The listing builds one solid part. Answer for the finished solid, in the listing's coordinates (mm). A direction names the side the tool comes from. Round coordinates to 2 decimals unless told otherwise and drop trailing zeros. Loops run counter-clockwise (first coordinate to the right, second up) from the corner with the lowest first, then second, coordinate; pieces in that order, holes last. Notation, with made-up numbers: (67, 76) -> (99, 76) arc R12 cw to (99, 98) -> close; hole circle Ø5 at (81, -5). An arc over 180 degrees is marked (long way). Answer in a Markdown table with one row per item. Add a question column.
```python
from build123d import *

# Parameters (mm, degrees)
SKETCH2_R                     = 3.811725635
F_18_TEETH_KNURLS_DEPTH       = 5.9944
SKETCH3_W                     = 1
SKETCH3_H                     = 6.35
CUT_EXTRUDE2_DEPTH            = 5.9944
SKETCH4_W                     = 9.4996
SKETCH4_H                     = 11.303
BODY_DEPTH                    = 7.0612
SKETCH6_W                     = 0.2286
SKETCH6_H                     = 0.7874
PINS_PTD901_ONE_SECTION_DEPTH = 3.5


with BuildPart() as part:
    # Sketch1 → Shaft Base (revolve)
    with BuildSketch(Plane.XY):
        Polygon((0, 3.5), (4.52755, 3.5), (5.0038, 3.02375), (5.0038, 0), (0, 0), align=None)
    revolve(axis=Axis((-1.517556918, 0, 0), (1, 0, 0)))

    # Sketch8 → K Style Shaft (revolve)
    with BuildSketch(Plane.XY):
        Polygon((5.0038, 3.00589629), (5.0038, 0), (15, 0), (15, 2.01414629), (14.0348, 2.97934629), (9.0056, 2.97934629), (9.0056, 2.01414629), (6.5024, 2.01414629), (5.51065, 3.00589629), align=None)
    revolve(axis=Axis((-8.258778459, 0, 0), (1, 0, 0)))

    # Sketch2 → 18 Teeth Knurls (cut)
    with BuildSketch(Plane(origin=(15, 0, 0), x_dir=(0, 0, -1), z_dir=(1, 0, 0))):
        Circle(SKETCH2_R)
        Polygon((0, 2.97934629), (0.353893751, 2.007031199), (1.018996445, 2.799669723), (1.018996445, 1.764953616), (1.91508688, 2.282311669), (1.561193129, 1.309996578), (2.580189574, 1.489673145), (1.91508688, 0.69703462), (2.934083325, 0.517358054), (2.03799289, 0), (2.934083325, -0.517358054), (1.91508688, -0.69703462), (2.580189574, -1.489673145), (1.561193129, -1.309996578), (1.91508688, -2.282311669), (1.018996445, -1.764953616), (1.018996445, -2.799669723), (0.353893751, -2.007031199), (0, -2.97934629), (-0.353893751, -2.007031199), (-1.018996445, -2.799669723), (-1.018996445, -1.764953616), (-1.91508688, -2.282311669), (-1.561193129, -1.309996578), (-2.580189574, -1.489673145), (-1.91508688, -0.69703462), (-2.934083325, -0.517358054), (-2.03799289, 0), (-2.934083325, 0.517358054), (-1.91508688, 0.69703462), (-2.580189574, 1.489673145), (-1.561193129, 1.309996578), (-1.91508688, 2.282311669), (-1.018996445, 1.764953616), (-1.018996445, 2.799669723), (-0.353893751, 2.007031199), align=None, mode=Mode.SUBTRACT)
    extrude(amount=-F_18_TEETH_KNURLS_DEPTH, mode=Mode.SUBTRACT)

    # Sketch3 → Cut-Extrude2 (cut)
    with BuildSketch(Plane(origin=(15, 0, 0), x_dir=(0, 0, -1), z_dir=(1, 0, 0))):
        Rectangle(SKETCH3_W, SKETCH3_H)
    extrude(amount=-CUT_EXTRUDE2_DEPTH, mode=Mode.SUBTRACT)

    # Sketch4 → Body (add)
    with BuildSketch(Plane.ZY):
        with Locations((0, -0.8509)):
            Rectangle(SKETCH4_W, SKETCH4_H)
    extrude(amount=BODY_DEPTH)

    # Sketch6 → Pins PTD901 (one section) (add)
    with BuildSketch(Plane.XZ.offset(6.5024)):
        with Locations((-5, -2.5)):
            Rectangle(SKETCH6_W, SKETCH6_H)
        with Locations((-5, 0)):
            Rectangle(SKETCH6_W, SKETCH6_H)
        with Locations((-5, 2.5)):
            Rectangle(SKETCH6_W, SKETCH6_H)
    extrude(amount=PINS_PTD901_ONE_SECTION_DEPTH)


solid = part.part
```
Item 1: The mould has two halves that part along Y. Classify faces 3 (the flat face through (15, 0, 1)), 4 (the flat face through (12.033, 0.606, 2.432)): +Y half, -Y half, draft (parallel to the pull), parting line (faces both ways), or undercut.
Item 2: Section A-A, the plane y = -8.75 is taken. Write down the section's boundary in (x, z).
Item 3: Flat-ended cylindrical pins translate along their axes: P1, Ø0.8, axis at x = 11, y = -2.5, coming from the -Z side; P2, Ø0.6, axis at y = -9, z = 0, coming from the -X side; P3, Ø4, axis at x = 6.5, y = -4, coming from the +Z side. Find the tip coordinate at first contact, or state that the pin passes through.
Item 4: Consider L1, parallel to Z at x = 11.25, y = -2; L2, parallel to X at y = -0.5, z = 3.5; L3, parallel to X at y = -2.25, z = -0.75. Determine where each line is inside the solid, lowest interval first. Write a range as from..to.
Item 5: Section D-D, the plane x = 1 is taken. Write down the section's boundary in (y, z), and give its area (3 significant figures).
Item 6: For faces 1 (the flat face through (9.006, 0, 0)), 2 (the flat face through (-3, -1, -4.75)), determine the directions among +Z, -Z, +X, -X, +Y, -Y from which every point of the face is accessible in a straight line to the end or side of a thin tool.
Here are the results:
| question | item | result |
|---|---|---|
| 1 | face 3 | draft |
| 1 | face 4 | undercut |
| 2 | outline | (-5.11, -2.89) -> (-4.89, -2.89) -> (-4.89, -2.11) -> (-5.11, -2.11) -> close; (-5.11, -0.39) -> (-4.89, -0.39) -> (-4.89, 0.39) -> (-5.11, 0.39) -> close; (-5.11, 2.11) -> (-4.89, 2.11) -> (-4.89, 2.89) -> (-5.11, 2.89) -> close |
| 3 | P1 | stops at z = -1.92 |
| 3 | P2 | stops at x = -5.11 |
| 3 | P3 | stops at z = 1.98 |
| 4 | L1 | z = -1.81..-1.43, -1.02..-0.5, 0.5..1.02, 1.43..1.81 |
| 4 | L2 | x = -7.06..0 |
| 4 | L3 | x = -7.06..6.14, 9.01..14.64 |
| 5 | outline | circle Ø7 at (0, 0) |
| 5 | area | 38.5 mm² |
| 6 | face 1 | +X, +Y, -Y |
| 6 | face 2 | -Z, +X, -X, +Y, -Y |
